Geometry: final body of the model. Coordinates: model frame, mm. Face numbers are marked on the shaded views. A direction names the side the tool comes from. Coordinates: 2 decimals unless noted, no trailing zeros. Write each loop counter-clockwise with the first axis right and the second up, starting at its lowest first coordinate (ties: lowest second). Pieces come first, ordered by that corner, then holes.
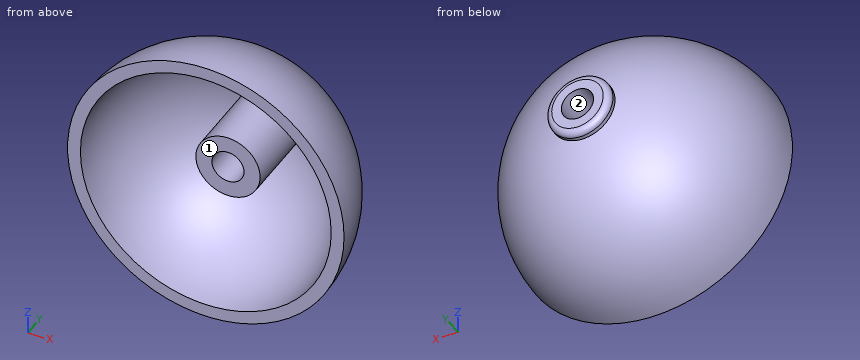
from build123d import *

# Parameters (mm, degrees)
SHELL1_T                 = -2
BOSS_EXTRUDE6_DEPTH      = 1
BOSS_EXTRUDE6_DEPTH_BACK = 15
SKETCH4_R                = 5
SKETCH2_R                = 2.5
CUT_EXTRUDE3_DEPTH       = 38.825256113
FILLET1_R                = 1


with BuildPart() as part:
    # Sketch1 → Revolve1 (revolve)
    with BuildSketch(Plane.XY):
        with BuildLine():
            Line((0, 0), (21.5, 0))
            ThreePointArc((21.5, 0), (15.202795796, 15.202795796), (0, 21.5))
            Line((0, 21.5), (0, 0))
        make_face()
    revolve(axis=Axis((0, 0, 0), (0, 1, 0)))

    # Shell1
    shell1_openings = [part.faces().sort_by_distance(p)[0] for p in [
        (0, 0, 0),
    ]]
    offset(amount=SHELL1_T, openings=shell1_openings, kind=Kind.INTERSECTION)

    # Sketch4 → Boss-Extrude6 (add, two sides: drawn at the far end of the back side and taken through both)
    with BuildSketch(Plane(origin=(0, 21.5, 0), x_dir=(1, 0, 0), z_dir=(0, 1, 0)).offset(-BOSS_EXTRUDE6_DEPTH_BACK)):
        with Locations(Location((0, 0, 0), (0, 0, 270))):
            Circle(SKETCH4_R)
    extrude(amount=BOSS_EXTRUDE6_DEPTH + BOSS_EXTRUDE6_DEPTH_BACK)

    # Sketch2 → Cut-Extrude3 (cut, through all)
    with BuildSketch(Plane(origin=(0, 0, 0), x_dir=(1, 0, 0), z_dir=(0, 1, 0))):
        with Locations(Location((0, 0, 0), (0, 0, 90))):
            Circle(SKETCH2_R)
    extrude(amount=CUT_EXTRUDE3_DEPTH, mode=Mode.SUBTRACT)

    # Fillet1
    fillet1_edges = [part.edges().sort_by_distance(p)[0] for p in [
        (0, 22.5, -5),
    ]]
    fillet(fillet1_edges, radius=FILLET1_R)


solid = part.part
Item 1: Section C-C, the plane y = 14.25. Output: boundary loops of the cut face in (x, z), plus the area to 3 significant figures.
Derived:
outline: circle Ø32.2 at (0, 0); circle Ø10 at (0, 0); hole circle Ø26.62 at (0, 0); hole circle Ø5 at (0, 0)
area: 317 mm2
Item 2: Set-up query: the marked faces 1 and 2. Return all of +Z, -Z, +X, -X, +Y, -Y with unobstructed straight access to the full face (end or side cutting, diameter ignored); none if empty.
Derived:
face 1: -Y
face 2: +Y, -Y
Item 3: Pin query (flat end, axial travel): pin 1 (3 mm diameter, centred on x = 0, z = 0, fed in from +Y); pin 2 (6 mm diameter, centred on x = -12, z = 8.5, fed in from +Y); pin 3 (6 mm diameter, centred on x = -7, y = 6, fed in from +Z); pin 4 (1.5 mm diameter, centred on y = 10, z = 2, fed in from -X). Return the tip coordinate at first contact, or that it passes through.
Derived:
pin 1: passes through
pin 2: stops at y = 18.03
pin 3: stops at z = 20.58
pin 4: stops at x = -19.31
Item 4: Section B-B, the plane z = 0. Output: boundary loops of the cut face in (x, y).
Derived:
outline: (-21.5, 0) - (-19.5, 0) arc R19.5 cw to (-5, 18.85) - (-5, 6.5) - (-2.5, 6.5) - (-2.5, 22.5) - (-4, 22.5) arc R1 ccw to (-5, 21.5) - (-5, 20.91) arc R21.5 ccw to start; (2.5, 6.5) - (5, 6.5) - (5, 18.85) arc R19.5 cw to (19.5, 0) - (21.5, 0) arc R21.5 ccw to (5, 20.91) - (5, 21.5) arc R1 ccw to (4, 22.5) - (2.5, 22.5) - close
Item 5: Section D-D, the plane y = 4. Output: boundary loops of the cut face in (x, z), plus the area to 3 significant figures.
Derived:
outline: circle Ø42.25 at (0, 0); hole circle Ø38.17 at (0, 0)
area: 258 mm2
Item 6: Material intervals for probe 1 along X at (y, z) = (15, 0); probe 2 along Z at (x, y) = (3, 16.75); probe 3 along Z at (x, y) = (-3.5, 16.75), sorted ascending.
Derived:
probe 1: x = -15.4 to -12.46, -5 to -2.5, 2.5 to 5, 12.46 to 15.4
probe 2: z = -13.14 to -9.52, -4 to 4, 9.52 to 13.14
probe 3: z = -13.02 to -9.35, -3.57 to 3.57, 9.35 to 13.02
Item 7: Section A-A, the plane x = 0. Output: boundary loops of the cut face in (y, z), plus the area to 3 significant figures.
Derived:
outline: (0, -21.5) arc R21.5 ccw to (20.91, -5) - (21.5, -5) arc R1 ccw to (22.5, -4) - (22.5, -2.5) - (6.5, -2.5) - (6.5, -5) - (18.85, -5) arc R19.5 cw to (0, -19.5) - close; (0, 19.5) arc R19.5 cw to (18.85, 5) - (6.5, 5) - (6.5, 2.5) - (22.5, 2.5) - (22.5, 4) arc R1 ccw to (21.5, 5) - (20.91, 5) arc R21.5 ccw to (0, 21.5) - close
area: 188 mm2
